The model under review builds one solid part; all positions refer to its coordinate system, in mm. A direction names the side the tool comes from. Round coordinates to 2 decimals unless told otherwise and drop trailing zeros. Order: outer loops, then holes, each group sorted by start corner. A loop starts at its lowest first (then second) coordinate and runs counter-clockwise, first axis right, second up.
Autodesk Inventor part; units mm, degrees
ref_plane "YZ Plane" through (0, 0, 0) normal (1, 0, 0) x (0, 1, 0)
ref_plane "XZ Plane" through (0, 0, 0) normal (0, 1, 0) x (-1, 0, 0)
ref_plane "XY Plane" through (0, 0, 0) normal (0, 0, 1) x (1, 0, 0)
sketch "Sketch1" plane through (0, 0, 0) normal (0, 1, 0) x (-1, 0, 0)
  line L0 (-6.3389, 5.775) -> (11.1611, 5.775)
  line L1 (11.1611, 5.775) -> (11.1611, -11.725)
  line L2 (11.1611, -11.725) -> (-6.3389, -11.725)
  line L3 (-6.3389, -11.725) -> (-6.3389, 5.775)
  point P0 (0, 0)
  dimension "d0" = 17.5
  dimension "d1" = 17.5
extrude "Extrusion1" add sketch "Sketch1" along normal blind 2.36
sketch "Sketch2" plane through (0, 2.36, 0) normal (0, 1, 0) x (1, 0, 0)
  circle A0 centre (-2.4111, 2.975) radius 4.3815
  point P0 (0, 0)
  dimension "d4" = 8.763
extrude "Extrusion2" add sketch "Sketch2" along normal blind 13.52
fillet "Fillet1" radius 3.175 4 edges at (6.3389, 1.18, 5.775) (-11.1611, 1.18, 5.775) (6.3389, 1.18, -11.725) (-11.1611, 1.18, -11.725)
properties part number "BNC_Up"
(1) Consider section A-A (x = -0.5). Write out the cut boundary in (y, z) (3 decimals).
Data:
outline: (0, -11.725) - (2.36, -11.725) - (2.36, -6.918) - (15.88, -6.918) - (15.88, 0.968) - (2.36, 0.968) - (2.36, 5.775) - (0, 5.775) - close
(2) Consider section B-B (z = -1.75). Write out the cut boundary in (x, y), and give its area (3 significant figures).
Data:
outline: (-11.16, 0) - (6.34, 0) - (6.34, 2.36) - (1.8, 2.36) - (1.8, 15.88) - (-6.62, 15.88) - (-6.62, 2.36) - (-11.16, 2.36) - close
area: 155 mm2
(3) Insertion check: pin 1 (8 mm diameter, centred on y = 6.5, z = -8, fed in from +X); pin 2 (3 mm diameter, centred on x = 2.5, y = 5, fed in from -Z); pin 3 (5 mm diameter, centred on x = -6, y = 10, fed in from -Z). Each pin has a flat end and moves straight along its axis. Give the tip position at first contact, or say it passes through.
Data:
pin 1: stops at x = 1.85
pin 2: stops at z = -5.72
pin 3: stops at z = -7.22
(4) For faces 1 (the flat face through (0, 2.36, 1)), 2 (the flat face through (-11.161, 1, -3)), list the 3-axis set-ups (+Z, -Z, +X, -X, +Y, -Y) from which the entire face can be reached by the end or side of a thin tool; tool diameter is ignored.
Data:
face 1: +Y
face 2: +Z, -Z, -X, +Y, -Y
(5) Consider section D-D (y = 10). Write out the cut boundary in (x, z) (1 decimal), and give its area (3 significant figures).
Data:
outline: circle Ø8.8 at (-2.4, -3)
area: 60.3 mm2
(6) Consider section C-C (x = 2.5). Write out the cut boundary in (y, z) (3 decimals), and give its area (3 significant figures).
Data:
outline: (0, -11.725) - (2.36, -11.725) - (2.36, 5.775) - (0, 5.775) - close
area: 41.3 mm2
(7) To check wall thickness, follow probe 1 along Y at (x, z) = (3.75, -4.5); probe 2 along X at (y, z) = (1, -8.75); probe 3 along X at (y, z) = (12.5, -6.25). State the ranges of each line that lie inside material, in increasing order.
Data:
probe 1: y = 0 to 2.36
probe 2: x = -11.15 to 6.33
probe 3: x = -5.32 to 0.5
